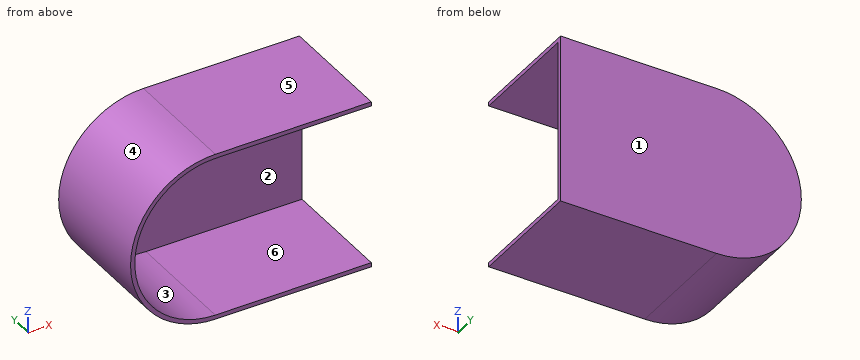
```python
from build123d import *

# Parameters (mm, degrees)
F1_DEPTH = 70
F2_T     = -2.5


with BuildPart() as f1:
    # F0 (on Front) → F1 (new body)
    with BuildSketch(Plane.XZ):
        with BuildLine():
            Line((-34.637429, 57.968741), (-126.637429, 57.968741))
            ThreePointArc((-126.637429, 57.968741), (-176.637429, 7.968741), (-126.637429, -42.031259))
            Line((-126.637429, -42.031259), (-34.637429, -42.031259))
            Line((-34.637429, -42.031259), (-34.637429, 57.968741))
        make_face()
    extrude(amount=F1_DEPTH)

    # F2
    f2_openings = [f1.faces().sort_by_distance(p)[0] for p in [
        (-34.637429, -35, 7.968741),
        (-100.746753, -70, 7.968741),
    ]]
    offset(amount=F2_T, openings=f2_openings)


solid = f1.part
```
The listing builds one solid part. Answer for the finished solid, in the listing's coordinates (mm). Face numbers are marked on the shaded views. A direction names the side the tool comes from. Round coordinates to 2 decimals unless told otherwise and drop trailing zeros. Loops run counter-clockwise (first coordinate to the right, second up) from the corner with the lowest first, then second, coordinate; pieces in that order, holes last.
Q1. Given pin 1 Ø3 at (x, z) = (-90.5, 34.5) entering from -Y; pin 2 Ø5 at (y, z) = (-41, 2) entering from +X; pin 3 Ø2 at (y, z) = (-41.5, 16) entering from +X, each flat-ended and moving along its own axis, determine where each tip first touches the part or whether it passes through.
Q2. Which of the six approach directions +Z, -Z, +X, -X, +Y, -Y give full straight-line access (tool end or side, diameter ignored) to the marked faces 5 and 6?
Q3. Section D-D, the plane z = -26 is taken. Determine the outline of the cut face in (x, y), then the cut area to 3 significant figures.
Q4. Section C-C, the plane z = 19.5 is taken. Determine the outline of the cut face in (x, y).
Q5. For a pull along Z with two mould halves and no side action, classify the marked faces 1, 2, 3 and 4 as released by +Z, released by -Z, zero draft, split by the parting line, or undercut.
Q6. Section A-A, the plane y = -58.5 is taken. Determine the outline of the cut face in (x, z).
Q7. Find the intervals of material crossed by line 1 (Z direction, x = -90, y = -7.5); line 2 (Y direction, x = -108, z = 44.5); line 3 (Z direction, x = -134, y = -51), in increasing order.
Q8. Section B-B, the plane x = -64.5 is taken. Determine the outline of the cut face in (y, z).
Completed:
1. pin 1: stops at y = -2.5
1. pin 2: stops at x = -173.38
1. pin 3: stops at x = -173.27
2. face 5: +Z, +X, -X, +Y, -Y
2. face 6: +X, -Y
3. outline: (-163.33, -70) - (-159.84, -70) - (-159.84, -2.5) - (-34.64, -2.5) - (-34.64, 0) - (-163.33, 0) - close
3. area: 557 mm2
4. outline: (-175.29, -70) - (-172.72, -70) - (-172.72, -2.5) - (-34.64, -2.5) - (-34.64, 0) - (-175.29, 0) - close
5. face 1: zero draft
5. face 2: undercut
5. face 3: undercut
5. face 4: split by the parting line
6. outline: (-126.64, -42.03) - (-34.64, -42.03) - (-34.64, -39.53) - (-126.64, -39.53) arc R47.5 cw to (-126.64, 55.47) - (-34.64, 55.47) - (-34.64, 57.97) - (-126.64, 57.97) arc R50 ccw to start
7. line 1: z = -42.03 to -39.53, 55.47 to 57.97
7. line 2: y = -2.5 to 0
7. line 3: z = -41.49 to -38.96, 54.89 to 57.42
8. outline: (-70, -42.03) - (0, -42.03) - (0, 57.97) - (-70, 57.97) - (-70, 55.47) - (-2.5, 55.47) - (-2.5, -39.53) - (-70, -39.53) - close
